Build history of the part. All positions in model axes, mm. A direction names the side the tool comes from. Give positions to 0.01 mm unless a question says otherwise; leave off trailing zeros. Order: outer loops, then holes, each group sorted by start corner. A loop starts at its lowest first (then second) coordinate and runs counter-clockwise, first axis right, second up. Notation, with made-up numbers: (14.5, 75) - (28.5, 75) arc R19 cw to (28.5, 104) - close; hole circle Ø5 at (51.5, -28). An arc over 180 degrees is marked (long way). One line per item, written item: value.
```python
from build123d import *

# Parameters (mm, degrees)
BOSS_EXTRUDE1_DEPTH = 8
BOSS_EXTRUDE2_START = 8
SKETCH3_7_W         = 139.5
SKETCH3_7_H         = 11.9
BOSS_EXTRUDE2_DEPTH = 15
FILLET1_R           = 8
CUT_EXTRUDE1_REACH  = 139.901
BOSS_EXTRUDE3_DEPTH = 12.5
BOSS_EXTRUDE4_DEPTH = 99.5
CUT_EXTRUDE3_REACH  = 138.81
SKETCH9_W           = 70
SKETCH9_H           = 11.9
SKETCH9_W_2         = 1
CUT_EXTRUDE5_REACH  = 139.901
SKETCH11_R          = 22
FILLET2_R           = 4
CUT_EXTRUDE6_REACH  = 139.342
SKETCH12_R          = 1.45
SKETCH13_R          = 4
CUT_EXTRUDE7_DEPTH  = 4
CUT_EXTRUDE2_REACH  = 232.432
SKETCH6_R           = 1.55


with BuildPart() as part:
    # Sketch3 → Boss-Extrude1 (new body)
    with BuildSketch(Plane(origin=(0, 0, 0), x_dir=(1, 0, 0), z_dir=(0, 1, 0))):
        with BuildLine():
            Line((-75, 110), (75, 110))
            ThreePointArc((75, 110), (78.535533906, 108.535533906), (80, 105))
            Line((80, 105), (80, -105))
            ThreePointArc((80, -105), (78.535533906, -108.535533906), (75, -110))
            Line((75, -110), (-75, -110))
            ThreePointArc((-75, -110), (-78.535533906, -108.535533906), (-80, -105))
            Line((-80, -105), (-80, 105))
            ThreePointArc((-80, 105), (-78.535533906, 108.535533906), (-75, 110))
        make_face()
    extrude(amount=BOSS_EXTRUDE1_DEPTH)

    # Sketch3<7> → Boss-Extrude2 (add)
    with BuildSketch(Plane(origin=(0, 0, 0), x_dir=(1, 0, 0), z_dir=(0, 1, 0)).offset(BOSS_EXTRUDE2_START)):
        with Locations((0, 98.95)):
            Rectangle(SKETCH3_7_W, SKETCH3_7_H)
    extrude(amount=BOSS_EXTRUDE2_DEPTH)

    # Fillet1
    # the kernel refuses this fillet: 8 mm, written as the material it takes off along each edge
    with BuildSketch(Plane(origin=(89.75, 23, -93), x_dir=(0, -1, 0), z_dir=(-1, 0, 0)), Plane(origin=(-89.75, 23, -104.9), x_dir=(0, -1, 0), z_dir=(1, 0, 0))) as fillet1_piece_1:
        with BuildLine():
            CenterArc((FILLET1_R, -FILLET1_R), FILLET1_R, 90, 90)
            Line((0, -FILLET1_R), (0, 0))
            Line((0, 0), (FILLET1_R, 0))
        make_face()
    extrude(amount=179.5, mode=Mode.SUBTRACT)

    # Sketch4 → Cut-Extrude1 (cut, up to next)
    with BuildSketch(Plane.XZ, mode=Mode.PRIVATE) as cut_extrude1_sk1:
        with BuildLine():
            Line((-55, 0), (55, 0))
            ThreePointArc((55, 0), (58.535533906, -1.464466094), (60, -5))
            Line((60, -5), (60, -35))
            ThreePointArc((60, -35), (58.535533906, -38.535533906), (55, -40))
            Line((55, -40), (-55, -40))
            ThreePointArc((-55, -40), (-58.535533906, -38.535533906), (-60, -35))
            Line((-60, -35), (-60, -5))
            ThreePointArc((-60, -5), (-58.535533906, -1.464466094), (-55, 0))
        make_face()
    cut_extrude1_tool1 = extrude(cut_extrude1_sk1.sketch, amount=-CUT_EXTRUDE1_REACH, mode=Mode.PRIVATE) & part.part
    add(cut_extrude1_tool1.solids().sort_by_distance((0, 0, -20))[0], mode=Mode.SUBTRACT)

    # Sketch5 → Boss-Extrude3 (add)
    with BuildSketch(Plane(origin=(0, 8, 0), x_dir=(1, 0, 0), z_dir=(0, 1, 0))):
        with BuildLine():
            ThreePointArc((-69.5, -104.5), (-73.035533906, -103.035533906), (-74.5, -99.5))
            Line((-74.5, -99.5), (-74.5, 29.5))
            ThreePointArc((-74.5, 29.5), (-73.035533906, 33.035533906), (-69.5, 34.5))
            Line((-69.5, 34.5), (-69.5, -99.5))
            Line((-69.5, -99.5), (69.5, -99.5))
            Line((69.5, -99.5), (69.5, 34.5))
            ThreePointArc((69.5, 34.5), (73.035533906, 33.035533906), (74.5, 29.5))
            Line((74.5, 29.5), (74.5, -99.5))
            ThreePointArc((74.5, -99.5), (73.035533906, -103.035533906), (69.5, -104.5))
            Line((69.5, -104.5), (-69.5, -104.5))
        make_face()
    extrude(amount=BOSS_EXTRUDE3_DEPTH)

    # Sketch8 → Boss-Extrude4 (add)
    with BuildSketch(Plane(origin=(0, 0, 99.5), x_dir=(-1, 0, 0), z_dir=(0, 0, -1))):
        with BuildLine():
            ThreePointArc((-31.313789331, 8), (-37.73637637, 11.944397261), (-40.25, 19.05))
            Line((-40.25, 19.05), (-54.25, 19.05))
            Line((-54.25, 19.05), (-54.25, 4.75))
            Line((-54.25, 4.75), (-28.95, 4.75))
            ThreePointArc((-28.95, 4.75), (-33.770529017, 5.586995135), (-38.026756028, 8))
            Line((-38.026756028, 8), (-31.313789331, 8))
        make_face()
        with BuildLine():
            ThreePointArc((40.25, 19.05), (37.73637637, 11.944397261), (31.313789331, 8))
            Line((31.313789331, 8), (38.026756028, 8))
            ThreePointArc((38.026756028, 8), (33.770529017, 5.586995135), (28.95, 4.75))
            Line((28.95, 4.75), (54.25, 4.75))
            Line((54.25, 4.75), (54.25, 19.05))
            Line((54.25, 19.05), (40.25, 19.05))
        make_face()
    extrude(amount=BOSS_EXTRUDE4_DEPTH)

    # Sketch9 → Cut-Extrude3 (cut, up to next)
    with BuildSketch(Plane(origin=(0, 8, 0), x_dir=(1, 0, 0), z_dir=(0, 1, 0)), mode=Mode.PRIVATE) as cut_extrude3_sk1:
        with Locations((0, 98.95)):
            Rectangle(SKETCH9_W, SKETCH9_H)
    cut_extrude3_tool1 = extrude(cut_extrude3_sk1.sketch, amount=CUT_EXTRUDE3_REACH, mode=Mode.PRIVATE) & part.part
    # Sketch9 → Cut-Extrude3 (cut, up to next)
    with BuildSketch(Plane(origin=(0, 8, 0), x_dir=(1, 0, 0), z_dir=(0, 1, 0)), mode=Mode.PRIVATE) as cut_extrude3_sk2:
        with Locations((-69.25, 98.95)):
            Rectangle(SKETCH9_W_2, SKETCH9_H)
    cut_extrude3_tool2 = extrude(cut_extrude3_sk2.sketch, amount=CUT_EXTRUDE3_REACH, mode=Mode.PRIVATE) & part.part
    # Sketch9 → Cut-Extrude3 (cut, up to next)
    with BuildSketch(Plane(origin=(0, 8, 0), x_dir=(1, 0, 0), z_dir=(0, 1, 0)), mode=Mode.PRIVATE) as cut_extrude3_sk3:
        with Locations((69.25, 98.95)):
            Rectangle(SKETCH9_W_2, SKETCH9_H)
    cut_extrude3_tool3 = extrude(cut_extrude3_sk3.sketch, amount=CUT_EXTRUDE3_REACH, mode=Mode.PRIVATE) & part.part
    add(cut_extrude3_tool1.solids().sort_by_distance((0, 8, -98.95))[0], mode=Mode.SUBTRACT)
    add(cut_extrude3_tool2.solids().sort_by_distance((-69.25, 8, -98.95))[0], mode=Mode.SUBTRACT)
    add(cut_extrude3_tool3.solids().sort_by_distance((69.25, 8, -98.95))[0], mode=Mode.SUBTRACT)

    # Sketch11 → Cut-Extrude5 (cut, up to next)
    with BuildSketch(Plane.XZ, mode=Mode.PRIVATE) as cut_extrude5_sk1:
        with Locations(Location((0, -64.78, 0), (0, 0, 270))):
            Circle(SKETCH11_R)
    cut_extrude5_tool1 = extrude(cut_extrude5_sk1.sketch, amount=-CUT_EXTRUDE5_REACH, mode=Mode.PRIVATE) & part.part
    add(cut_extrude5_tool1.solids().sort_by_distance((0, 0, -64.78))[0], mode=Mode.SUBTRACT)

    # Fillet2
    fillet2_edges = [part.edges().sort_by_distance(p)[0] for p in [
        (54.25, 8, 49.75),
        (-54.25, 8, 49.75),
    ]]
    fillet(fillet2_edges, radius=FILLET2_R)

    # Sketch12 → Cut-Extrude6 (cut, up to next)
    with BuildSketch(Plane(origin=(0, 19.05, 0), x_dir=(1, 0, 0), z_dir=(0, 1, 0)), mode=Mode.PRIVATE) as cut_extrude6_sk1:
        with Locations(Location((48.25, -20, 0), (0, 0, 270))):
            Circle(SKETCH12_R)
    cut_extrude6_tool1 = extrude(cut_extrude6_sk1.sketch, amount=-CUT_EXTRUDE6_REACH, mode=Mode.PRIVATE) & part.part
    # Sketch12 → Cut-Extrude6 (cut, up to next)
    with BuildSketch(Plane(origin=(0, 19.05, 0), x_dir=(1, 0, 0), z_dir=(0, 1, 0)), mode=Mode.PRIVATE) as cut_extrude6_sk2:
        with Locations(Location((-48.25, -79.5, 0), (0, 0, 270))):
            Circle(SKETCH12_R)
    cut_extrude6_tool2 = extrude(cut_extrude6_sk2.sketch, amount=-CUT_EXTRUDE6_REACH, mode=Mode.PRIVATE) & part.part
    add(cut_extrude6_tool1.solids().sort_by_distance((48.25, 19.05, 20))[0], mode=Mode.SUBTRACT)
    add(cut_extrude6_tool2.solids().sort_by_distance((-48.25, 19.05, 79.5))[0], mode=Mode.SUBTRACT)

    # Sketch13 → Cut-Extrude7 (cut)
    with BuildSketch(Plane.XZ):
        with Locations(Location((-48.25, 79.5, 0), (0, 0, 270))):
            Circle(SKETCH13_R)
        with Locations(Location((48.25, 20, 0), (0, 0, 270))):
            Circle(SKETCH13_R)
    extrude(amount=-CUT_EXTRUDE7_DEPTH, mode=Mode.SUBTRACT)

    # Sketch6 → Cut-Extrude2 (cut, up to next)
    with BuildSketch(Plane(origin=(0, 0, -104.9), x_dir=(-1, 0, 0), z_dir=(0, 0, -1)), mode=Mode.PRIVATE) as cut_extrude2_sk1:
        with Locations((-51.875, 11.5)):
            Circle(SKETCH6_R)
    cut_extrude2_tool1 = extrude(cut_extrude2_sk1.sketch, amount=-CUT_EXTRUDE2_REACH, mode=Mode.PRIVATE) & part.part
    # Sketch6 → Cut-Extrude2 (cut, up to next)
    with BuildSketch(Plane(origin=(0, 0, -104.9), x_dir=(-1, 0, 0), z_dir=(0, 0, -1)), mode=Mode.PRIVATE) as cut_extrude2_sk2:
        with Locations(Location((51.875, 11.5, 0), (0, 0, 180))):
            Circle(SKETCH6_R)
    cut_extrude2_tool2 = extrude(cut_extrude2_sk2.sketch, amount=-CUT_EXTRUDE2_REACH, mode=Mode.PRIVATE) & part.part
    add(cut_extrude2_tool1.solids().sort_by_distance((51.875, 11.5, -104.9))[0], mode=Mode.SUBTRACT)
    add(cut_extrude2_tool2.solids().sort_by_distance((-51.875, 11.5, -104.9))[0], mode=Mode.SUBTRACT)


solid = part.part
```
(1) Pin check, flat tips, straight feed: P1, Ø3.5, axis at x = 48.25, z = 20, coming from the +Y side; P2, Ø1.5, axis at x = 48.5, z = -60.5, coming from the +Y side; P3, Ø8, axis at x = 43.5, z = -34.5, coming from the +Y side; P4, Ø2.5, axis at x = -50, z = 80.5, coming from the -Y side. Stop position of each tip, or through.
Completed:
P1: y = 19.05
P2: y = 8
P3: through
P4: y = 4
(2) Slice it at B-B, the plane z = 32. Give the cut face in (x, y), and give its area (3 significant figures).
Completed:
outline: (-80, 0) - (80, 0) - (80, 8) - (74.5, 8) - (74.5, 20.5) - (69.5, 20.5) - (69.5, 8) - (58.25, 8) arc R4 cw to (54.25, 12) - (54.25, 19.05) - (40.25, 19.05) arc R11.3 cw to (31.31, 8) - (-31.31, 8) arc R11.3 cw to (-40.25, 19.05) - (-54.25, 19.05) - (-54.25, 12) arc R4 cw to (-58.25, 8) - (-69.5, 8) - (-69.5, 20.5) - (-74.5, 20.5) - (-74.5, 8) - (-80, 8) - close
area: 1,770 mm²
(3) Drill centre lines: line 1 (Z direction, x = 60, y = 11.75); line 2 (X direction, y = 15.75, z = 20); line 3 (X direction, y = 2.4, z = 20). Where is each one in solid material? Low to high.
Completed:
line 1: -104.9 to -93, 99.5 to 104.5
line 2: -74.5 to -69.5, -54.25 to -39.76, 39.76 to 46.8, 49.7 to 54.25, 69.5 to 74.5
line 3: -80 to 44.25, 52.25 to 80
(4) Slice it at C-C, the plane z = -52. Give the cut face in (x, y).
Completed:
outline: (-80, 0) - (-17.91, 0) - (-17.91, 8) - (-80, 8) - close; (17.91, 0) - (80, 0) - (80, 8) - (17.91, 8) - close
(5) Pull direction Z, two halves, no side cores. Call faces 4 (the face through (74.5, 14, 34)), 5 (the face through (-60, 4, -20)), 6 (the face through (78, 4, -109)): +Z half, -Z half, draft (parallel to the pull), parting line (faces both ways), or undercut.
Completed:
face 4: draft
face 5: undercut
face 6: -Z half
(6) Slice it at A-A, the plane x = 0. Give the cut face in (y, z).
Completed:
outline: (0, -110) - (8, -110) - (8, -86.78) - (0, -86.78) - close; (0, -42.78) - (8, -42.78) - (8, -40) - (0, -40) - close; (0, 0) - (8, 0) - (8, 99.5) - (20.5, 99.5) - (20.5, 104.5) - (8, 104.5) - (8, 110) - (0, 110) - close
(7) 3-axis set-ups, long thin cutter, end or side, ignore diameter. For faces 1 (the face through (52, 9, -104.9)), 2 (the face through (-54.25, 15, 50)), 3 (the face through (-69.5, 14, 32)): which of +Z, -Z, +X, -X, +Y, -Y reach the whole face in a straight line?
Completed:
face 1: -Z, +X, -X, +Y
face 2: +Y
face 3: -Z, +Y
